Autodesk Inventor part; units mm, degrees
ref_plane "YZ Plane" through (0, 0, 0) normal (1, 0, 0) x (0, 1, 0)
ref_plane "XZ Plane" through (0, 0, 0) normal (0, 1, 0) x (-1, 0, 0)
ref_plane "XY Plane" through (0, 0, 0) normal (0, 0, 1) x (1, 0, 0)
sketch "Sketch1" plane through (0, 0, 0) normal (0, 0, 1) x (1, 0, 0)
  line L0 (-490, 50) -> (490, 50)
  line L1 (490, 50) -> (490, 0)
  line L2 (490, 0) -> (-490, 0)
  line L3 (-490, 0) -> (-490, 50)
  point P0 (0, 0)
  point P1 (0, 0)
  dimension "d0" = 980
  dimension "d1" = 50
extrude "Plate1" add sketch "Sketch1" along normal blind 2
sketch "Sketch2" plane through (490, 2, 0) normal (0, -1, 0) x (1, 0, 0)
  line L0 (-980, 0) -> (0, 0)
  line L1 (0, 0) -> (0, 20)
  line L2 (0, 20) -> (-980, 20)
  line L3 (-980, 20) -> (-980, 0)
edge flange "Flange1" height 20 angle 90 thickness 2 bend radius 2.75 thickness toward (0, -1, 0) relief tear relief width 2 relief depth 1 edges at (0, 0, 2) wall of the first edge with corners at (-490, 2, 0) (490, 2, 0) (490, 2, 20) (-490, 2, 20)
bend "Bend1"
corner "Corner1"
sketch "Sketch5" plane through (0, 0, 0) normal (0, 0, -1) x (-1, 0, 0)
  line L0 (490, 50) -> (-490, 50)
  line L1 (490, 0) -> (-490, 0)
  circle A0 centre (0, 50) radius 30
  line L2 (-490, 0) -> (-490, 50)
  line L3 (490, 0) -> (490, 50)
  circle A1 centre (-490, 50) radius 30
  circle A2 centre (490, 50) radius 30
  line L4 (-246, 50) -> (-244, 50)
  line L5 (-244, 50) -> (-244, 21)
  line L6 (-244, 21) -> (-246, 21)
  line L7 (-246, 21) -> (-246, 50)
  line L8 (244, 50) -> (246, 50)
  line L9 (246, 50) -> (246, 21)
  line L10 (246, 21) -> (244, 21)
  line L11 (244, 21) -> (244, 50)
  line L12 (0, 50) -> (0, 0) construction
  point P0 (245, 21)
  point P1 (-245, 21)
  point P2 (-490, 20)
  point P3 (-460, 50)
  point P4 (-30, 50)
  point P5 (30, 50)
  point P6 (460, 50)
  point P7 (490, 20)
  point P8 (-244, 50)
  point P9 (246, 50)
  dimension "d33" = 60
  dimension "d34" = 2
  dimension "d35" = 29
  dimension "d36" = 490
extrude "Extrusion1" cut sketch "Sketch5" against normal through all contours L9 L10 L11 L0 | L0 L3 A2 | A0 L0 | L5 L6 L7 L0 | L2 L0 A1 picked at (470.2507, 47.7748) picked at (6.5355, 34.7298) picked at (-470.2507, 47.7748)
sketch "Sketch7" plane through (0, 0, 2) normal (0, 0, 1) x (1, 0, 0)
  line L0 (468.7934, 20.88) -> (468.7934, 8.88) construction
  line L1 (468.7934, 8.88) -> (251.3453, 8.88) construction
  line L2 (251.3453, 8.88) -> (251.3453, 20.88) construction
  line L3 (251.3453, 20.88) -> (468.7934, 20.88) construction
  line L4 (-244, 50) -> (-30, 50)
  point P0 (0, 0)
  point P1 (-1, 50)
  point P2 (1, 50)
  dimension "d30" = 12
mark "Mark1"
equation "\"d1\" = Стрингер_7"
equation "\"d2\" = Thickness"
equation "\"d3\" = BendReliefWidth"
equation "\"d4\" = BendReliefDepth"
equation "\"d5\" = MinimumRemnant"
equation "\"d6\" = TransitionRadius"
equation "\"d9\" = BendRadius"
equation "\"d10\" = CornerReliefSize"
equation "\"d11\" = GapSize"
equation "\"d12\" = JacobiRadiusSize"
equation "\"GapSize\" = Thickness"
equation "\"MinimumRemnant\" = 2 * Thickness"
equation "\"BendReliefDepth\" = 0.5 * Thickness"
equation "\"BendReliefWidth\" = Thickness"
equation "\"CornerReliefSize\" = 4 * Thickness"
equation "\"JacobiRadiusSize\" = BendRadius"
equation "\"TransitionRadius\" = BendRadius"
equation "\"Стрингер_7\" = 50"
properties part number "MSC 504 STRINGER BOARD BELLY" material "Stainless Steel"
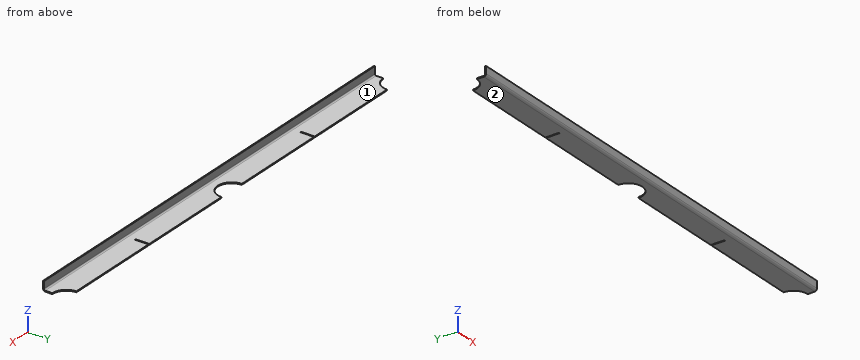
CAD build for the part. Positions are in the model's coordinates, mm. Face numbers are marked on the shaded views. A direction names the side the tool comes from. Give positions to 0.01 mm unless a question says otherwise; leave off trailing zeros. Order: outer loops, then holes, each group sorted by start corner. A loop starts at its lowest first (then second) coordinate and runs counter-clockwise, first axis right, second up. Notation, with made-up numbers: (56.5, 54) - (102.5, 54) arc R19 cw to (102.5, 75) - close; hole circle Ø8 at (36, 79). An arc over 180 degrees is marked (long way). Answer in a Markdown table with one row per item.
1. Saw through at B-B, the plane x = 0. Give the cut face in (y, z).
Data:
| item | result |
|---|---|
| outline | (0, 4.75) arc R4.75 ccw to (4.75, 0) - (20, 0) - (20, 2) - (4.75, 2) arc R2.75 cw to (2, 4.75) - (2, 20) - (0, 20) - close |
2. Probe probe 1 along Z at (x, y) = (286.5, 20); probe 2 along X at (y, z) = (33.5, 1.25). List the from-to ranges inside material, lowest first. Write a range as [from, to].
Data:
| item | result |
|---|---|
| probe 1 | z = [0, 2] |
| probe 2 | x = [-464.95, -246], [-244, -25.05], [25.05, 244], [246, 464.95] |
3. Tool access for the marked faces 1 and 2: list every direction of +Z, -Z, +X, -X, +Y, -Y with a clear straight run to the whole face (end or side of a thin tool).
Data:
| item | result |
|---|---|
| face 1 | +Z, +X, -X, +Y |
| face 2 | -Z, +X, -X, +Y, -Y |
4. Saw through at C-C, the plane z = 13.25. Give the cut face in (x, y), plus the area to 3 significant figures.
Data:
| item | result |
|---|---|
| outline | (-490, 0) - (490, 0) - (490, 2) - (-490, 2) - close |
| area | 1,960 mm² |
5. Saw through at A-A, the plane y = 31. Give the cut face in (x, z).
Data:
| item | result |
|---|---|
| outline | (-466.78, 0) - (-246, 0) - (-246, 2) - (-466.78, 2) - close; (-244, 0) - (-23.22, 0) - (-23.22, 2) - (-244, 2) - close; (23.22, 0) - (244, 0) - (244, 2) - (23.22, 2) - close; (246, 0) - (466.78, 0) - (466.78, 2) - (246, 2) - close |
6. Flat gauge pins, fed straight in: pin 1 (0.6 mm diameter, centred on x = -245.5, z = 0.5, fed in from +Y); pin 2 (5 mm diameter, centred on x = -21, z = 2, fed in from -Y); pin 3 (5 mm diameter, centred on x = -161.5, y = 26, fed in from +Z). Where does each tip first touch, or does it go through?
Data:
| item | result |
|---|---|
| pin 1 | stops at y = 21 |
| pin 2 | stops at y = 0.01 |
| pin 3 | stops at z = 2 |
